The model under review builds one solid part; all positions refer to its coordinate system, in mm. Face numbers are marked on the shaded views. A direction names the side the tool comes from. Give positions to 0.01 mm unless a question says otherwise; leave off trailing zeros. Order: outer loops, then holes, each group sorted by start corner. A loop starts at its lowest first (then second) coordinate and runs counter-clockwise, first axis right, second up. Notation, with made-up numbers: (70, 23) - (128, 23) arc R10 ccw to (128, 40) - close; hole circle Ø4 at (35, 37). An arc over 180 degrees is marked (long way). Put each result on its own line as item: value.
```python
from build123d import *

# Parameters (mm, degrees)
SKETCH001_R  = 8.55
PAD001_DEPTH = 5
SKETCH002_R  = 8.574514
PAD_DEPTH    = 4


with BuildPart() as part:
    # Sketch001 → Pad001 (new body)
    with BuildSketch(Plane.XY):
        Polygon((21.45, -48.595033), (10.725, -30.018788), (-10.725, -30.018788), (-21.45, -48.595033), (-10.725, -67.171278), (10.725, -67.171278), align=None)
        with Locations((0, -48.595033)):
            Circle(SKETCH001_R, mode=Mode.SUBTRACT)
    extrude(amount=PAD001_DEPTH)

    # Sketch002 → Pad (join)
    with BuildSketch(Plane.XY.offset(5)):
        Polygon((23.5, -48.619546), (11.75, -28.267949), (-11.75, -28.267949), (-23.5, -48.619546), (-11.75, -68.971143), (11.75, -68.971143), align=None)
        with Locations((0, -48.619546)):
            Circle(SKETCH002_R, mode=Mode.SUBTRACT)
    extrude(amount=PAD_DEPTH)


solid = part.part
```
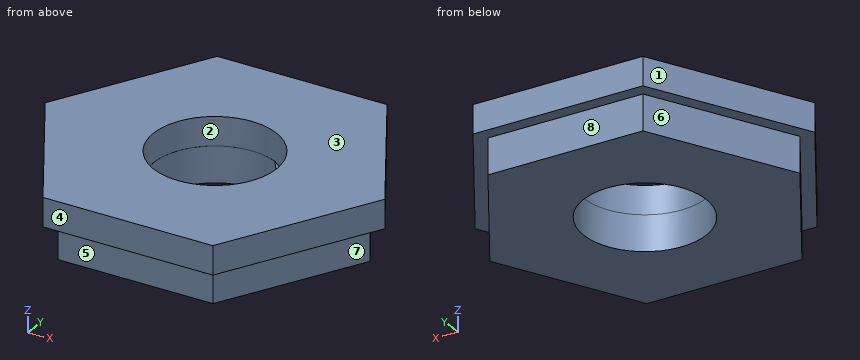
(1) Take a section at A-A, the plane z = 4.25. Write out the cut boundary in (x, y) (3 decimals), then the cut area to 3 significant figures.
The answers:
outline: (-21.45, -48.595) - (-10.725, -67.171) - (10.725, -67.171) - (21.45, -48.595) - (10.725, -30.019) - (-10.725, -30.019) - close; hole circle Ø17.1 at (0, -48.595)
area: 966 mm^2
(2) Take a section at C-C, the plane y = -54.5. Write out the cut boundary in (x, z).
The answers:
outline: (-20.1, 5) - (-18.04, 5) - (-18.04, 0) - (-6.18, 0) - (-6.18, 5) - (-6.24, 5) - (-6.24, 9) - (-20.1, 9) - close; (6.18, 0) - (18.04, 0) - (18.04, 5) - (20.1, 5) - (20.1, 9) - (6.24, 9) - (6.24, 5) - (6.18, 5) - close
(3) For the marked faces 4, 5, 6, 7 and 8, list the 3-axis set-ups (+Z, -Z, +X, -X, +Y, -Y) from which the entire face can be reached by the end or side of a thin tool; tool diameter is ignored.
The answers:
face 4: +Z, -Z, +X, -X, -Y
face 5: -Z, +X, -X, -Y
face 6: -Z, -X, +Y
face 7: -Z, +X, -Y
face 8: -Z, +X, -X, +Y
(4) Clearance check with flat-ended pins moving along their axes: pin 1 Ø1 at (y, z) = (-52, 6) entering from -X; pin 2 Ø8.5 at (x, y) = (1.5, -52) entering from +Z. State where each tip first meets the part, or that it passes through.
The answers:
pin 1: x = -21.84
pin 2: through
(5) Take a section at D-D, the plane z = 7.25. Write out the cut boundary in (x, y), then the cut area to 3 significant figures.
The answers:
outline: (-23.5, -48.62) - (-11.75, -68.97) - (11.75, -68.97) - (23.5, -48.62) - (11.75, -28.27) - (-11.75, -28.27) - close; hole circle Ø17.15 at (0, -48.62)
area: 1,200 mm^2
(6) The part is to be moulded in two halves that separate along Y. For the marked faces 1, 2 and 3, say which applies: pulls with the +Y half, pulls with the -Y half, needs draft (parallel to the pull), parting line crosses it, or undercut.
The answers:
face 1: pulls with the +Y half
face 2: undercut
face 3: needs draft
(7) Wall thickness on L1, parallel to Y at x = 0, z = 3.1; L2, parallel to Y at x = 0, z = 8.5; L3, parallel to X at y = -52.5, z = 0.75: over which ranges is each line inside the solid? List them lowest first.
The answers:
L1: -67.17 to -57.15, -40.05 to -30.02
L2: -68.97 to -57.19, -40.05 to -28.27
L3: -19.2 to -7.61, 7.61 to 19.2
